Verification items for this drawing (mm, ordinates from the low corner). A direction names the side the tool comes from. Coordinates: 2 decimals unless noted, no trailing zeros. Write each loop counter-clockwise with the first axis right and the second up, starting at its lowest first coordinate (ties: lowest second). Pieces come first, ordered by that corner, then holes.
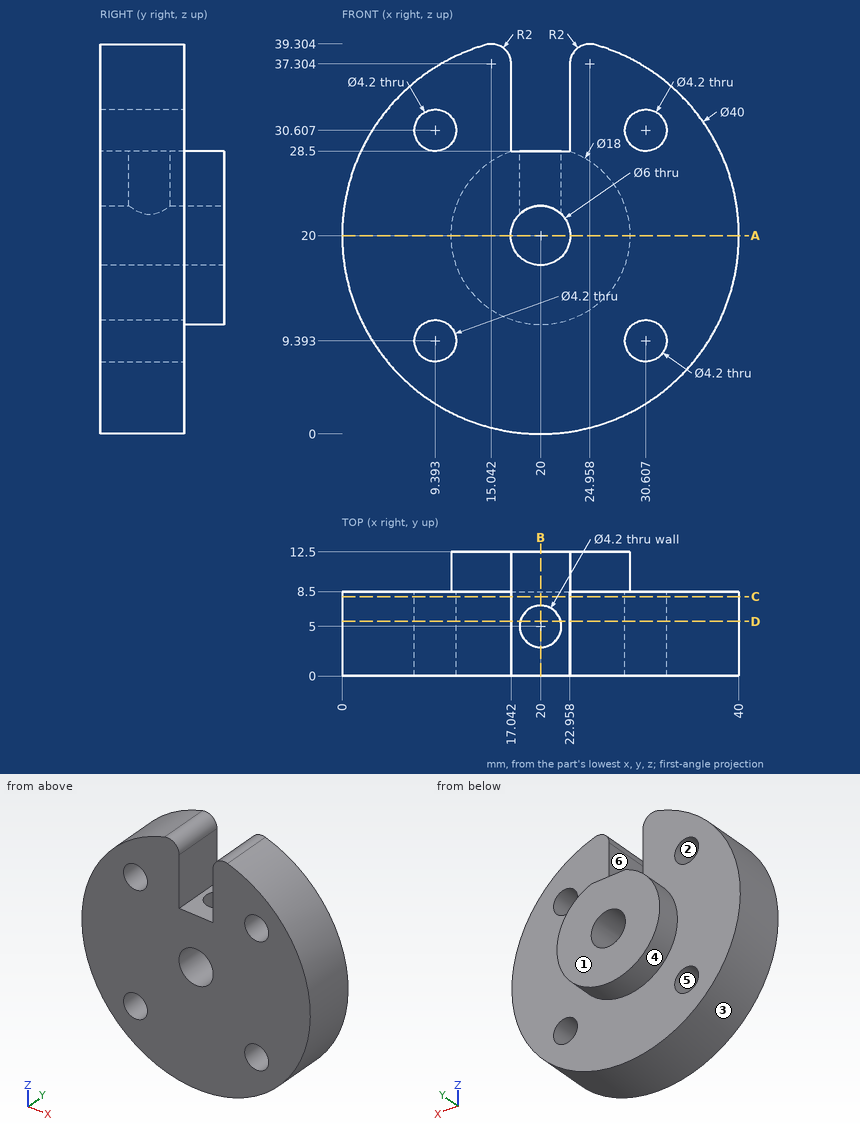
1. Access from +Z, -Z, +X, -X, +Y, -Y to the whole of each face (thin tool, end or side, straight path). Record for the marked faces 4, 5 and 6.
Computed values:
face 4: +Y
face 5: +Y, -Y
face 6: +Z, +Y, -Y
2. Thickness scan on line 1 along Z through (x, y) = (29.5, 3.25); line 2 along Z through (x, y) = (30.5, 3.25) (1 decimal); line 3 along Y through (x, z) = (7, 8). Record the ranges inside material, lowest first.
Computed values:
line 1: z = 2.4 to 7.61, 11.18 to 28.82, 32.39 to 37.6
line 2: z = 3 to 7.3, 11.5 to 28.5, 32.7 to 37
line 3: y = 0 to 8.5
3. Draft check along X on the marked faces 1, 2 and 3. Enter one of: released by +X, released by -X, zero draft, split by the parting line, or undercut.
Computed values:
face 1: zero draft
face 2: undercut
face 3: split by the parting line
4. Sectioned sample at D-D, the plane y = 5.5. Record the boundary of the cut face in (x, z), and give its area (3 significant figures).
Computed values:
outline: (14.49, 39.23) arc R20 ccw (long way) to (25.51, 39.23) arc R2 ccw to (22.96, 37.3) - (22.96, 28.5) - (22.04, 28.5) - (22.04, 22.2) arc R3 cw (long way) to (17.96, 22.2) - (17.96, 28.5) - (17.04, 28.5) - (17.04, 37.3) arc R2 ccw to start; hole circle Ø4.2 at (9.39, 9.39); hole circle Ø4.2 at (9.39, 30.61); hole circle Ø4.2 at (30.61, 9.39); hole circle Ø4.2 at (30.61, 30.61)
area: 1,080 mm2
5. Sectioned sample at A-A, the plane z = 20. Record the boundary of the cut face in (x, y).
Computed values:
outline: (0, 0) - (17, 0) - (17, 12.5) - (11, 12.5) - (11, 8.5) - (0, 8.5) - close; (23, 0) - (40, 0) - (40, 8.5) - (29, 8.5) - (29, 12.5) - (23, 12.5) - close
6. Sectioned sample at C-C, the plane y = 8. Record the boundary of the cut face in (x, z), and give its area (3 significant figures).
Computed values:
outline: (14.49, 39.23) arc R20 ccw (long way) to (25.51, 39.23) arc R2 ccw to (22.96, 37.3) - (22.96, 28.5) - (17.04, 28.5) - (17.04, 37.3) arc R2 ccw to start; hole circle Ø4.2 at (9.39, 9.39); hole circle Ø4.2 at (9.39, 30.61); hole circle Ø6 at (20, 20); hole circle Ø4.2 at (30.61, 9.39); hole circle Ø4.2 at (30.61, 30.61)
area: 1,100 mm2
7. Gauge pin test, flat ends, axial feed: pin 1 Ø6 at (x, z) = (32, 24.5) entering from +Y; pin 2 Ø7 at (y, z) = (6, 34) entering from +X; pin 3 Ø3 at (x, y) = (19, 9) entering from +Z. Record the tip position at first contact, or that the pin passes through.
Computed values:
pin 1: stops at y = 8.5
pin 2: stops at x = 37.02
pin 3: stops at z = 28.5
8. Sectioned sample at B-B, the plane x = 20. Record the boundary of the cut face in (y, z).
Computed values:
outline: (0, 0) - (8.5, 0) - (8.5, 11) - (12.5, 11) - (12.5, 17) - (0, 17) - close; (0, 23) - (2.9, 23) - (2.9, 28.5) - (0, 28.5) - close; (7.1, 23) - (12.5, 23) - (12.5, 28.5) - (7.1, 28.5) - close
